Here's how the part is built. I have some questions about the finished solid (model axes, mm). Face numbers are marked on the shaded views. A direction names the side the tool comes from. Round coordinates to 2 decimals unless told otherwise and drop trailing zeros. Loops run counter-clockwise (first coordinate to the right, second up) from the corner with the lowest first, then second, coordinate; pieces in that order, holes last. Notation, with made-up numbers: (8.5, 52) -> (36.5, 52) arc R19 ccw to (36.5, 65) -> close; hole circle Ø9 at (-24, 58). An arc over 180 degrees is marked (long way). Use one line per item in the form item = value. Start each with the question number.
Item 1: I'm going to push flat-ended pins straight in: pin 1 Ø4.5 at (x, y) = (64, -10) entering from +Z; pin 2 Ø11.5 at (x, z) = (0, 35) entering from +Y (3 decimals); pin 3 Ø6 at (y, z) = (-11, 38.5) entering from -X; pin 4 Ø1.7 at (x, y) = (-64, -10) entering from -Z. Where does each tip first touch, or does it pass through?
Item 2: If we section it at B-B (z = 35): Write out the boundary of the cut face in (x, y) (3 decimals).
Item 3: For the marked faces 1, 2 and 3, which set-ups out of +Z, -Z, +X, -X, +Y, -Y let a thin tool reach every point of the face, with its end or its side?
Item 4: If I drill on L1, parallel to Y at x = -64, z = -1.4; L2, parallel to Y at x = 16, z = 9.5; L3, parallel to X at y = 1.75, z = 35, over which ranges is the centre line in solid material (lowest first)? Write a range as [from, to].
Item 5: If we section it at D-D (y = 5): Write out the boundary of the cut face in (x, z), then the cut area to 3 significant figures.
Item 6: If we section it at A-A (x = -64): Write out the boundary of the cut face in (y, z), then the cut area to 3 significant figures.
Item 7: If we section it at C-C (x = 0): Write out the boundary of the cut face in (y, z) (3 decimals), then the cut area to 3 significant figures.
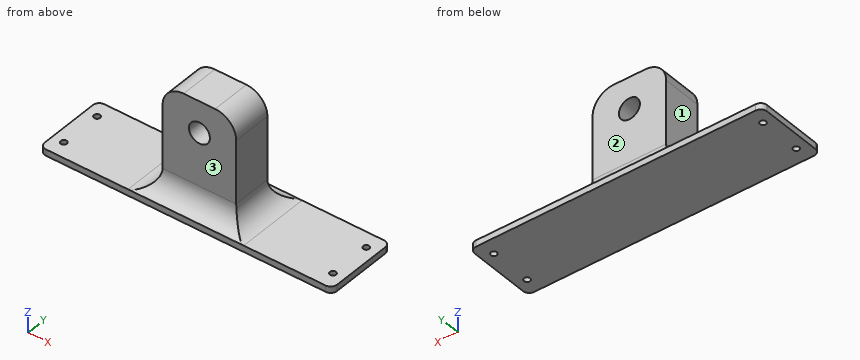
```python
from build123d import *

# Parameters (mm, degrees)
ESQUISSE7_W             = 139
ESQUISSE7_H             = 35
BOSS_EXTRU_1_DEPTH      = 3
ESQUISSE8_W             = 35
ESQUISSE8_H             = 18.75
BOSS_EXTRU_2_DEPTH      = 50
CONG_1_R                = 10
D_GAGEMENT_M2_52_D      = 2.9
ESQUISSE9_R             = 5
ENL_V_MAT_EXTRU_2_DEPTH = 90.73581019
CONG_2_R                = 3


with BuildPart() as part:
    # Esquisse7 → Boss.-Extru.1 (new body)
    with BuildSketch(Plane.XY):
        Rectangle(ESQUISSE7_W, ESQUISSE7_H)
    extrude(amount=-BOSS_EXTRU_1_DEPTH)

    # Esquisse8 → Boss.-Extru.2 (add)
    with BuildSketch(Plane.XY):
        Rectangle(ESQUISSE8_W, ESQUISSE8_H)
    extrude(amount=BOSS_EXTRU_2_DEPTH)

    # Congé1
    # the kernel refuses this fillet: 10 mm, written as the material it adds along each edge
    with BuildSketch(Plane(origin=(17.5, 9.375, 0), x_dir=(1, 0, 0), z_dir=(0, -1, 0)), Plane(origin=(-17.5, -9.375, 0), x_dir=(-1, 0, 0), z_dir=(0, 1, 0))) as cong_1_piece_1:
        with BuildLine():
            CenterArc((CONG_1_R, CONG_1_R), CONG_1_R, 180, 90)
            Line((0, CONG_1_R), (0, 0))
            Line((0, 0), (CONG_1_R, 0))
        make_face()
    extrude(amount=18.75)
    with BuildSketch(Plane(origin=(-17.5, 9.375, 0), x_dir=(0, 1, 0), z_dir=(1, 0, 0)), Plane(origin=(17.5, -9.375, 0), x_dir=(0, -1, 0), z_dir=(-1, 0, 0))) as cong_1_piece_2:
        with BuildLine():
            CenterArc((10, 9.822646028), CONG_1_R, 180, 79.193077125)
            Line((0, 9.822646028), (0, 0))
            Line((0, 0), (8.125, 0))
        make_face()
    extrude(amount=35)
    with BuildSketch(Plane(origin=(-17.5, 9.375, 0), x_dir=(0, 1, 0), z_dir=(1, 0, 0))) as cong_1_piece_3a_section:
        with BuildLine():
            CenterArc((10, 9.822646028), CONG_1_R, 180, 79.193077125)
            Line((0, 9.822646028), (0, 0))
            Line((0, 0), (8.125, 0))
        make_face()
    cong_1_piece_3a = extrude(amount=59.556615071, mode=Mode.PRIVATE)
    cong_1_piece_3a = split(cong_1_piece_3a, bisect_by=Plane(origin=(17.5, 9.375, 0), z_dir=(1, 0, 0)), keep=Keep.TOP, mode=Mode.PRIVATE)
    with BuildSketch(Plane(origin=(17.5, 34.375, 0), x_dir=(1, 0, 0), z_dir=(0, -1, 0))) as cong_1_piece_3b_section:
        with BuildLine():
            CenterArc((CONG_1_R, CONG_1_R), CONG_1_R, 180, 90)
            Line((0, CONG_1_R), (0, 0))
            Line((0, 0), (CONG_1_R, 0))
        make_face()
    cong_1_piece_3b = extrude(amount=43.75, mode=Mode.PRIVATE)
    cong_1_piece_3b = split(cong_1_piece_3b, bisect_by=Plane(origin=(17.5, 17.5, 0), z_dir=(0, -1, 0)), keep=Keep.TOP, mode=Mode.PRIVATE)
    cong_1_piece_3b = split(cong_1_piece_3b, bisect_by=Plane(origin=(17.5, 9.375, 0), z_dir=(0, 1, 0)), keep=Keep.TOP, mode=Mode.PRIVATE)
    cong_1_piece_3 = cong_1_piece_3a & cong_1_piece_3b
    add(cong_1_piece_3)
    with BuildSketch(Plane(origin=(17.5, 9.375, 0), x_dir=(1, 0, 0), z_dir=(0, -1, 0))) as cong_1_piece_4a_section:
        with BuildLine():
            CenterArc((CONG_1_R, CONG_1_R), CONG_1_R, 180, 90)
            Line((0, CONG_1_R), (0, 0))
            Line((0, 0), (CONG_1_R, 0))
        make_face()
    cong_1_piece_4a = extrude(amount=43.75, mode=Mode.PRIVATE)
    cong_1_piece_4a = split(cong_1_piece_4a, bisect_by=Plane(origin=(17.5, -17.5, 0), z_dir=(0, 1, 0)), keep=Keep.TOP, mode=Mode.PRIVATE)
    cong_1_piece_4a = split(cong_1_piece_4a, bisect_by=Plane(origin=(17.5, -9.375, 0), z_dir=(0, -1, 0)), keep=Keep.TOP, mode=Mode.PRIVATE)
    with BuildSketch(Plane(origin=(42.056615071, -9.375, 0), x_dir=(0, -1, 0), z_dir=(-1, 0, 0))) as cong_1_piece_4b_section:
        with BuildLine():
            CenterArc((10, 9.822646028), CONG_1_R, 180, 79.193077125)
            Line((0, 9.822646028), (0, 0))
            Line((0, 0), (8.125, 0))
        make_face()
    cong_1_piece_4b = extrude(amount=59.556615071, mode=Mode.PRIVATE)
    cong_1_piece_4b = split(cong_1_piece_4b, bisect_by=Plane(origin=(17.5, -9.375, 0), z_dir=(1, 0, 0)), keep=Keep.TOP, mode=Mode.PRIVATE)
    cong_1_piece_4 = cong_1_piece_4a & cong_1_piece_4b
    add(cong_1_piece_4)
    with BuildSketch(Plane(origin=(-42.056615071, 9.375, 0), x_dir=(0, 1, 0), z_dir=(1, 0, 0))) as cong_1_piece_5a_section:
        with BuildLine():
            CenterArc((10, 9.822646028), CONG_1_R, 180, 79.193077125)
            Line((0, 9.822646028), (0, 0))
            Line((0, 0), (8.125, 0))
        make_face()
    cong_1_piece_5a = extrude(amount=59.556615071, mode=Mode.PRIVATE)
    cong_1_piece_5a = split(cong_1_piece_5a, bisect_by=Plane(origin=(-17.5, 9.375, 0), z_dir=(-1, 0, 0)), keep=Keep.TOP, mode=Mode.PRIVATE)
    with BuildSketch(Plane(origin=(-17.5, -9.375, 0), x_dir=(-1, 0, 0), z_dir=(0, 1, 0))) as cong_1_piece_5b_section:
        with BuildLine():
            CenterArc((CONG_1_R, CONG_1_R), CONG_1_R, 180, 90)
            Line((0, CONG_1_R), (0, 0))
            Line((0, 0), (CONG_1_R, 0))
        make_face()
    cong_1_piece_5b = extrude(amount=43.75, mode=Mode.PRIVATE)
    cong_1_piece_5b = split(cong_1_piece_5b, bisect_by=Plane(origin=(-17.5, 17.5, 0), z_dir=(0, -1, 0)), keep=Keep.TOP, mode=Mode.PRIVATE)
    cong_1_piece_5b = split(cong_1_piece_5b, bisect_by=Plane(origin=(-17.5, 9.375, 0), z_dir=(0, 1, 0)), keep=Keep.TOP, mode=Mode.PRIVATE)
    cong_1_piece_5 = cong_1_piece_5a & cong_1_piece_5b
    add(cong_1_piece_5)
    with BuildSketch(Plane(origin=(17.5, -9.375, 0), x_dir=(0, -1, 0), z_dir=(-1, 0, 0))) as cong_1_piece_6a_section:
        with BuildLine():
            CenterArc((10, 9.822646028), CONG_1_R, 180, 79.193077125)
            Line((0, 9.822646028), (0, 0))
            Line((0, 0), (8.125, 0))
        make_face()
    cong_1_piece_6a = extrude(amount=59.556615071, mode=Mode.PRIVATE)
    cong_1_piece_6a = split(cong_1_piece_6a, bisect_by=Plane(origin=(-17.5, -9.375, 0), z_dir=(-1, 0, 0)), keep=Keep.TOP, mode=Mode.PRIVATE)
    with BuildSketch(Plane(origin=(-17.5, -34.375, 0), x_dir=(-1, 0, 0), z_dir=(0, 1, 0))) as cong_1_piece_6b_section:
        with BuildLine():
            CenterArc((CONG_1_R, CONG_1_R), CONG_1_R, 180, 90)
            Line((0, CONG_1_R), (0, 0))
            Line((0, 0), (CONG_1_R, 0))
        make_face()
    cong_1_piece_6b = extrude(amount=43.75, mode=Mode.PRIVATE)
    cong_1_piece_6b = split(cong_1_piece_6b, bisect_by=Plane(origin=(-17.5, -17.5, 0), z_dir=(0, 1, 0)), keep=Keep.TOP, mode=Mode.PRIVATE)
    cong_1_piece_6b = split(cong_1_piece_6b, bisect_by=Plane(origin=(-17.5, -9.375, 0), z_dir=(0, -1, 0)), keep=Keep.TOP, mode=Mode.PRIVATE)
    cong_1_piece_6 = cong_1_piece_6a & cong_1_piece_6b
    add(cong_1_piece_6)
    # the kernel refuses this fillet: 10 mm, written as the material it takes off along each edge
    with BuildSketch(Plane(origin=(17.5, 34.375, 50), x_dir=(-1, 0, 0), z_dir=(0, -1, 0))) as cong_1_2_piece_1:
        with BuildLine():
            CenterArc((CONG_1_R, CONG_1_R), CONG_1_R, 180, 90)
            Line((0, CONG_1_R), (0, 0))
            Line((0, 0), (CONG_1_R, 0))
        make_face()
    extrude(amount=68.75, mode=Mode.SUBTRACT)
    with BuildSketch(Plane(origin=(-17.5, -34.375, 50), x_dir=(0, 0, -1), z_dir=(0, 1, 0))) as cong_1_2_piece_2:
        with BuildLine():
            CenterArc((CONG_1_R, -CONG_1_R), CONG_1_R, 90, 90)
            Line((0, -CONG_1_R), (0, 0))
            Line((0, 0), (CONG_1_R, 0))
        make_face()
    extrude(amount=68.75, mode=Mode.SUBTRACT)

    # Dégagement M2.52 (through all)
    with Locations(Plane.XY):
        with Locations((64, -10), (64, 10), (-64, -10), (-64, 10)):
            Hole(D_GAGEMENT_M2_52_D / 2)

    # Esquisse9 → Enlèv. mat.-Extru.2 (cut, through all)
    with BuildSketch(Plane(origin=(0, -9.375, 0), x_dir=(-1, 0, 0), z_dir=(0, -1, 0))):
        with Locations(Location((0, -35, 0), (0, 0, 90))):
            Circle(ESQUISSE9_R)
    extrude(amount=-ENL_V_MAT_EXTRU_2_DEPTH, mode=Mode.SUBTRACT)

    # Congé2
    cong_2_edges = [part.edges().sort_by_distance(p)[0] for p in [
        (-69.5, 17.5, -1.5),
        (69.5, 17.5, -1.5),
        (69.5, -17.5, -1.5),
        (-69.5, -17.5, -1.5),
    ]]
    fillet(cong_2_edges, radius=CONG_2_R)


solid = part.part
```
Values found:
q1.pin_1 = 0
q1.pin_2 = 9.375
q1.pin_3 = -17.5
q1.pin_4 = through
q2.outline = (-17.5, -9.375) -> (-5, -9.375) -> (-5, 9.375) -> (-17.5, 9.375) -> close; (5, -9.375) -> (17.5, -9.375) -> (17.5, 9.375) -> (5, 9.375) -> close
q3.face_1 = +Z, -X, +Y, -Y
q3.face_2 = +Z, +X, -X, +Y
q3.face_3 = +Z, +X, -X, -Y
q4.L1 = [-17.5, -11.45], [-8.55, 8.55], [11.45, 17.5]
q4.L2 = [-9.38, 9.38]
q4.L3 = [-17.5, -5], [5, 17.5]
q5.outline = (-69.5, -3) -> (69.5, -3) -> (69.5, 0) -> (27.5, 0) arc R10 cw to (17.5, 10) -> (17.5, 40) arc R10 ccw to (7.5, 50) -> (-7.5, 50) arc R10 ccw to (-17.5, 40) -> (-17.5, 10) arc R10 cw to (-27.5, 0) -> (-69.5, 0) -> close; hole circle Ø10 at (0, 35)
q5.area = 2,090 mm2
q6.outline = (-17.5, -3) -> (-11.45, -3) -> (-11.45, 0) -> (-17.5, 0) -> close; (-8.55, -3) -> (8.55, -3) -> (8.55, 0) -> (-8.55, 0) -> close; (11.45, -3) -> (17.5, -3) -> (17.5, 0) -> (11.45, 0) -> close
q6.area = 87.6 mm2
q7.outline = (-17.5, -3) -> (17.5, -3) -> (17.5, 0) arc R10 cw to (9.375, 9.823) -> (9.375, 30) -> (-9.375, 30) -> (-9.375, 9.823) arc R10 cw to (-17.5, 0) -> close; (-9.375, 40) -> (9.375, 40) -> (9.375, 50) -> (-9.375, 50) -> close
q7.area = 895 mm2
